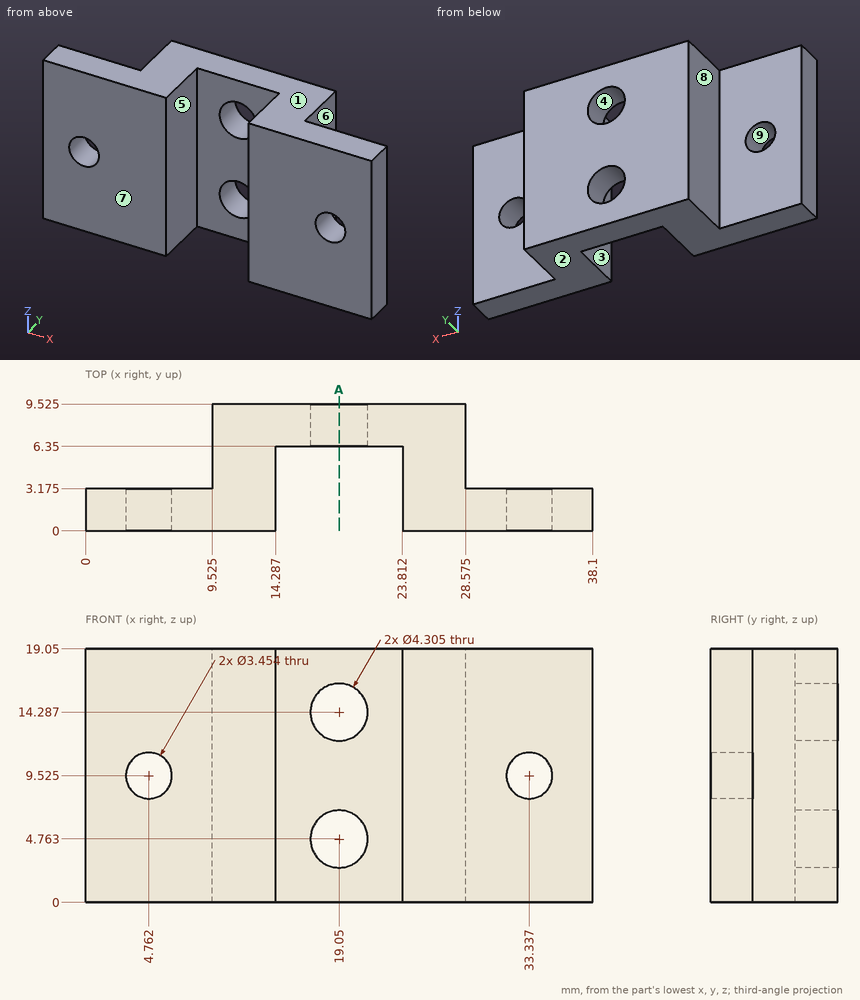
The figure shows three views and two pictorial views of one solid part (mm, origin at its lowest corner). Answer the questions. A direction names the side the tool comes from. Coordinates: 2 decimals unless noted, no trailing zeros. Write item = value, one per line. Start each with the question number.
1) The mould has two halves that part along Z. Classify the marked faces 1, 2, 3 and 4: released by +Z, released by -Z, zero draft, split by the parting line, or undercut.
2) A cutting plane is placed at A-A (x = 19.05). Count the separate pieces of the cut face and the enclosed holes in it.
3) A tool of negligible diameter and unlimited length cuts with its end or side. For the marked faces 5, 6, 7, 8 and 9, from which of +Z, -Z, +X, -X, +Y, -Y can it reach the whole face along a straight path? Write none if from no direction.
4) Straight lines are drawn through the part: line 1 (X direction, y = 1.5, z = 12.25); line 2 (X direction, y = 3.25, z = 7) (1 decimal); line 3 (X direction, y = 1.5, z = 10.75) (1 decimal). For each, find the intervals that lie inside material, in ascending order. Write a range as from..to.
5) Given pin 1 Ø1.9 at (y, z) = (6.5, 13) entering from +X (1 decimal); pin 2 Ø4 at (x, z) = (4.76, 9.52) entering from -Y; pin 3 Ø7.5 at (x, z) = (4.5, 10) entering from +Y (1 decimal); pin 4 Ø5 at (x, z) = (19.05, 4.76) entering from -Y, each flat-ended and moving along its own axis, determine where each tip first touches the part or whether it passes through.
Responses:
q1.face_1 = released by +Z
q1.face_2 = released by -Z
q1.face_3 = zero draft
q1.face_4 = undercut
q2.separate_pieces = 3
q2.enclosed_holes = 0
q3.face_5 = +Z, -Z, -Y
q3.face_6 = +Z, -Z, +X, +Y
q3.face_7 = +Z, -Z, +X, -X, -Y
q3.face_8 = +Z, -Z, -X, +Y
q3.face_9 = +Y, -Y
q4.line_1 = 0..14.29, 23.81..38.1
q4.line_2 = 9.5..14.3, 23.8..28.6
q4.line_3 = 0..3.5, 6..14.3, 23.8..32.1, 34.6..38.1
q5.pin_1 = 28.6
q5.pin_2 = 0
q5.pin_3 = 3.2
q5.pin_4 = 6.35
